Work out the finished part from the listing and answer in its coordinate system (mm). A direction names the side the tool comes from. Give positions to 0.01 mm unless a question says otherwise; leave off trailing zeros. Loops run counter-clockwise (first coordinate to the right, second up) from the corner with the lowest first, then second, coordinate; pieces in that order, holes last. Notation, with made-up numbers: (14, 12.25) -> (66, 12.25) arc R27 cw to (66, 46.25) -> close; hole circle Ø1 at (-2.75, -23). An arc over 180 degrees is marked (long way). Answer as CSV lines item,"result". Start each with the question number.
1. Find section A-A, the plane y = -23. Give the vertices of the cut face in (x, z), and give its area (3 significant figures).
2. Find section B-B, the plane x = 130. Give the vertices of the cut face in (y, z).
3. Flat-ended cylindrical pins translate along their axes: pin 1 Ø1.2 at (y, z) = (34.5, -0.5) entering from -X; pin 2 Ø1.2 at (y, z) = (39, 0.5) entering from +X; pin 3 Ø0.8 at (x, z) = (-51.5, 0.5) entering from -Y. Find the tip coordinate at first contact, or state that the pin passes through.
4. Find the intervals of material crossed by line 1 along X through (y, z) = (14, 1); line 2 along X through (y, z) = (1.5, -0.55); line 3 along Y through (x, z) = (121, -0.6), in increasing order.
5. Find section D-D, the plane x = 0. Give the vertices of the cut face in (y, z), and give its area (3 significant figures).
6. Determine the mould class of faces 1 (the face through (-38.391, -24.005, 0.018)), 2 (the face through (-16.1, 24, 0)), 3 (the face through (40, 1, 1.25)) for opening direction X: +X half, -X half, draft (parallel to the pull), parting line (faces both ways), or undercut.
7. A tool of negligible diameter and unlimited length cuts with its end or side. For faces 4 (the face through (8.666, 24.143, 0.018)), 5 (the face through (-29.35, 44.93, -0.02)), 6 (the face through (8.568, -24.045, 0.018)), from which of +Z, -Z, +X, -X, +Y, -Y can it reach the whole face along a straight path? Write none if from no direction.
8. Find section C-C, the plane z = -0.8. Count the separate pieces of the cut face and the enclosed holes in it, and give its area (3 significant figures).
from build123d import *

# Parameters (mm, degrees)
F0_R     = 2.8
F0_R_2   = 1.6
F0_R_3   = 1.5
F0_R_4   = 1
F1_DEPTH = 1.25


with BuildPart() as f1:
    # F0 (on Top) → F1 (new body, symmetric)
    with BuildSketch(Plane.XY):
        with BuildLine():
            Line((-67.989561, 18), (-67.989561, 0))
            Line((-67.989561, 0), (-67.989561, -18))
            ThreePointArc((-67.989561, -18), (-67.403774, -19.414214), (-65.989561, -20))
            Line((-65.989561, -20), (-43.224092, -20))
            ThreePointArc((-43.224092, -20), (-42.458725, -20.152241), (-41.809879, -20.585786))
            Line((-41.809879, -20.585786), (-34.875347, -27.520318))
            ThreePointArc((-34.875347, -27.520318), (-34.441802, -28.169165), (-34.289561, -28.934531))
            Line((-34.289561, -28.934531), (-34.289561, -43.035682))
            ThreePointArc((-34.289561, -43.035682), (-27.289561, -50.035682), (-20.289561, -43.035682))
            Line((-20.289561, -43.035682), (-20.289561, -29.015935))
            ThreePointArc((-20.289561, -29.015935), (-20.13732, -28.250568), (-19.703774, -27.601721))
            Line((-19.703774, -27.601721), (-12.687839, -20.585786))
            ThreePointArc((-12.687839, -20.585786), (-12.038993, -20.152241), (-11.273626, -20))
            Line((-11.273626, -20), (3.694504, -20))
            ThreePointArc((3.694504, -20), (4.459871, -20.152241), (5.108718, -20.585786))
            Line((5.108718, -20.585786), (12.124653, -27.601721))
            ThreePointArc((12.124653, -27.601721), (12.558198, -28.250568), (12.710439, -29.015935))
            Line((12.710439, -29.015935), (12.710439, -38))
            ThreePointArc((12.710439, -38), (13.296226, -39.414214), (14.710439, -40))
            Line((14.710439, -40), (150.010439, -40))
            ThreePointArc((150.010439, -40), (151.424653, -39.414214), (152.010439, -38))
            Line((152.010439, -38), (152.010439, 0))
            Line((152.010439, 0), (152.010439, 38))
            ThreePointArc((152.010439, 38), (151.424653, 39.414214), (150.010439, 40))
            Line((150.010439, 40), (14.710439, 40))
            ThreePointArc((14.710439, 40), (13.296226, 39.414214), (12.710439, 38))
            Line((12.710439, 38), (12.710439, 29.015935))
            ThreePointArc((12.710439, 29.015935), (12.558198, 28.250568), (12.124653, 27.601721))
            Line((12.124653, 27.601721), (5.108718, 20.585786))
            ThreePointArc((5.108718, 20.585786), (4.459871, 20.152241), (3.694504, 20))
            Line((3.694504, 20), (-11.273626, 20))
            ThreePointArc((-11.273626, 20), (-12.038993, 20.152241), (-12.687839, 20.585786))
            Line((-12.687839, 20.585786), (-19.703774, 27.601721))
            ThreePointArc((-19.703774, 27.601721), (-20.13732, 28.250568), (-20.289561, 29.015935))
            Line((-20.289561, 29.015935), (-20.289561, 43.035682))
            ThreePointArc((-20.289561, 43.035682), (-27.289561, 50.035682), (-34.289561, 43.035682))
            Line((-34.289561, 43.035682), (-34.289561, 28.106104))
            Line((-34.289561, 28.106104), (-41.809879, 20.585786))
            ThreePointArc((-41.809879, 20.585786), (-42.458725, 20.152241), (-43.224092, 20))
            Line((-43.224092, 20), (-65.989561, 20))
            ThreePointArc((-65.989561, 20), (-67.403774, 19.414214), (-67.989561, 18))
        make_face()
        with Locations((-27.289561, -43.035682)):
            Circle(F0_R, mode=Mode.SUBTRACT)
        with Locations((-27.289561, -33.135682)):
            Circle(F0_R_2, mode=Mode.SUBTRACT)
        with Locations((-65.254413, -16.519763)):
            Circle(F0_R_3, mode=Mode.SUBTRACT)
        with Locations((-59.297452, -16.519763)):
            Circle(F0_R_3, mode=Mode.SUBTRACT)
        with Locations((-3.989561, -15)):
            Circle(F0_R_3, mode=Mode.SUBTRACT)
        with Locations((8.010439, -15)):
            Circle(F0_R_3, mode=Mode.SUBTRACT)
        with Locations((-37.09171, 0)):
            Circle(F0_R_4, mode=Mode.SUBTRACT)
        Polygon((-34.289561, 0), (-34.289561, 6.2), (-11.289561, 6.2), (-11.289561, 0), (-11.289561, -6.2), (-34.289561, -6.2), align=None, mode=Mode.SUBTRACT)
        with Locations((-65.254413, 16.519763)):
            Circle(F0_R_3, mode=Mode.SUBTRACT)
        with Locations((-59.297452, 16.519763)):
            Circle(F0_R_3, mode=Mode.SUBTRACT)
        with Locations((-8.59171, 0)):
            Circle(F0_R_4, mode=Mode.SUBTRACT)
        with Locations((-3.989561, 15)):
            Circle(F0_R_3, mode=Mode.SUBTRACT)
        with Locations((8.010439, 15)):
            Circle(F0_R_3, mode=Mode.SUBTRACT)
        with Locations((-27.289561, 33.135682)):
            Circle(F0_R_2, mode=Mode.SUBTRACT)
        with Locations((-27.289561, 43.035682)):
            Circle(F0_R, mode=Mode.SUBTRACT)
    extrude(amount=F1_DEPTH, both=True)


solid = f1.part
Resolved:
1,outline,"(-39.4, -1.25) -> (-15.1, -1.25) -> (-15.1, 1.25) -> (-39.4, 1.25) -> close; (7.52, -1.25) -> (152.01, -1.25) -> (152.01, 1.25) -> (7.52, 1.25) -> close"
1,area,"422 mm^2"
2,outline,"(-40, -1.25) -> (40, -1.25) -> (40, 1.25) -> (-40, 1.25) -> close"
3,pin 1,"stops at x = -34.29"
3,pin 2,"stops at x = 151.97"
3,pin 3,"stops at y = -20"
4,line 1,"x = -67.99 to -5.11, -2.87 to 6.89, 9.13 to 152.01"
4,line 2,"x = -67.99 to -34.29, -11.29 to 152.01"
4,line 3,"y = -40 to 40"
5,outline,"(-20, -1.25) -> (20, -1.25) -> (20, 1.25) -> (-20, 1.25) -> close"
5,area,"100 mm^2"
6,face 1,"-X half"
6,face 2,"undercut"
6,face 3,"draft"
7,face 4,"+Z, -Z, +Y"
7,face 5,"+Z, -Z"
7,face 6,"+Z, -Z, -Y"
8,separate pieces,"1"
8,enclosed holes,"15"
8,area,"15,000 mm^2"
